The listing builds one solid part. Answer for the finished solid, in the listing's coordinates (mm). Coordinates: 2 decimals unless noted, no trailing zeros. Write each loop counter-clockwise with the first axis right and the second up, starting at its lowest first coordinate (ties: lowest second). Pieces come first, ordered by that corner, then holes.
from build123d import *

# Parameters (mm, degrees)
SKETCH1_R           = 2.38125
BOSS_EXTRUDE1_DEPTH = 5.842
FILLET1_R           = 1.5875
FILLET2_R           = 6.35
FILLET3_R           = 1.5875
CUT_EXTRUDE1_DEPTH  = 122.916897323
FILLET4_R           = 3.175


with BuildPart() as part:
    # Sketch1 → Boss-Extrude1 (new body)
    with BuildSketch(Plane(origin=(0, 0, 0), x_dir=(1, 0, 0), z_dir=(0, 1, 0))):
        Polygon((-10.998522628, -6.35), (-23.207348419, 14.79630657), (-89.198484187, -23.30369343), (-82.848484187, -34.302216058), (-79.673484187, -39.801477372), (-85.172745501, -42.976477372), (-93.847006815, -40.652216058), (-106.547006815, -18.655170802), (-85.725, 40.19630657), (-20.751477372, 61.34261314), (10.998522628, 6.35), align=None)
        with Locations(Location((-28.575, 49.493351826, 0), (0, 0, 270))):
            Circle(SKETCH1_R, mode=Mode.SUBTRACT)
        with Locations(Location((-22.225, 38.494829198, 0), (0, 0, 270))):
            Circle(SKETCH1_R, mode=Mode.SUBTRACT)
        with Locations(Location((-15.875, 27.49630657, 0), (0, 0, 270))):
            Circle(SKETCH1_R, mode=Mode.SUBTRACT)
        with Locations(Location((-9.525, 16.497783942, 0), (0, 0, 270))):
            Circle(SKETCH1_R, mode=Mode.SUBTRACT)
        with Locations(Location((-3.175, 5.499261314, 0), (0, 0, 270))):
            Circle(SKETCH1_R, mode=Mode.SUBTRACT)
        with Locations(Location((-43.2397154, 27.49630657, 0), (0, 0, 270))):
            Circle(SKETCH1_R, mode=Mode.SUBTRACT)
        with Locations(Location((-55.9397154, 27.49630657, 0), (0, 0, 270))):
            Circle(SKETCH1_R, mode=Mode.SUBTRACT)
        with Locations(Location((-68.6397154, 27.49630657, 0), (0, 0, 270))):
            Circle(SKETCH1_R, mode=Mode.SUBTRACT)
        with Locations(Location((-81.3397154, 27.49630657, 0), (0, 0, 270))):
            Circle(SKETCH1_R, mode=Mode.SUBTRACT)
        Polygon((-37.872045256, 40.19630657), (-42.195906773, 47.685454402), (-65.206843197, 40.19630657), align=None, mode=Mode.SUBTRACT)
    extrude(amount=BOSS_EXTRUDE1_DEPTH)

    # Fillet1
    fillet1_edges = [part.edges().sort_by_distance(p)[0] for p in [
        (-42.195906773, 2.921, -47.685454402),
        (-65.206843197, 2.921, -40.19630657),
        (-37.872045256, 2.921, -40.19630657),
    ]]
    fillet(fillet1_edges, radius=FILLET1_R)

    # Fillet2
    fillet2_edges = [part.edges().sort_by_distance(p)[0] for p in [
        (-85.725, 2.921, -40.19630657),
        (-20.751477372, 2.921, -61.34261314),
        (-85.172745501, 2.921, 42.976477372),
        (-93.847006815, 2.921, 40.652216058),
        (-106.547006815, 2.921, 18.655170802),
    ]]
    fillet(fillet2_edges, radius=FILLET2_R)

    # Fillet3
    fillet3_edges = [part.edges().sort_by_distance(p)[0] for p in [
        (10.998522628, 2.921, -6.35),
        (-10.998522628, 2.921, 6.35),
        (-23.207348419, 2.921, -14.79630657),
        (-89.198484187, 2.921, 23.30369343),
        (-79.673484187, 2.921, 39.801477372),
    ]]
    fillet(fillet3_edges, radius=FILLET3_R)

    # Sketch2 → Cut-Extrude1 (cut, through all)
    with BuildSketch(Plane(origin=(0, 5.842, 0), x_dir=(1, 0, 0), z_dir=(0, 1, 0))):
        Polygon((-84.549961559, -5.955170802), (-48.607348419, 14.79630657), (-77.207963999, 14.79630657), align=None)
    extrude(amount=-CUT_EXTRUDE1_DEPTH, mode=Mode.SUBTRACT)

    # Fillet4
    fillet4_edges = [part.edges().sort_by_distance(p)[0] for p in [
        (-84.549961559, 2.921, 5.955170802),
        (-77.207963999, 2.921, -14.79630657),
        (-48.607348419, 2.921, -14.79630657),
    ]]
    fillet(fillet4_edges, radius=FILLET4_R)


solid = part.part
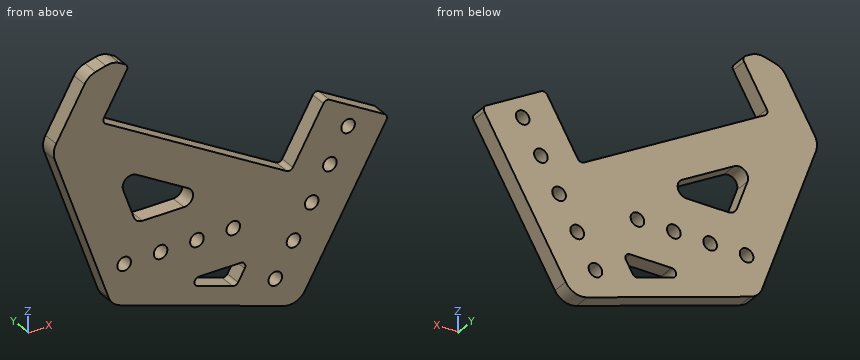
Q1. The part is cut by section C-C, the plane z = -50. Write down the section's boundary in (x, y).
Answers below:
outline: (-55.6, 0) - (-30.9, 0) - (-30.9, 5.84) - (-55.6, 5.84) - close; (-26.25, 0) - (-14.2, 0) - (-14.2, 5.84) - (-26.25, 5.84) - close
Q2. The part is cut by section A-A, the plane x = -63.5. Write down the section's boundary in (y, z).
Answers below:
outline: (0, -47.43) - (5.84, -47.43) - (5.84, -14.8) - (0, -14.8) - close; (0, -6.2) - (5.84, -6.2) - (5.84, 8.47) - (0, 8.47) - close
Q3. Find the intervals of material crossed by probe 1 along X at (y, z) = (2.25, -2); probe 2 along X at (y, z) = (5.05, -5); probe 3 along Z at (x, y) = (-85.5, 0.3), in increasing order.
Answers below:
probe 1: x = -99.24 to -81.73, -70.77 to -45.37, -15.82 to 3.46
probe 2: x = -98.18 to -80.67, -65.58 to -40.18, -17.55 to -5.5, -0.85 to 8.66
probe 3: z = -39.38 to 21.17, 29.71 to 42.49
Q4. The part is cut by section D-D, the plane y = 4.9. State how many separate pieces and enclosed holes the cut face has, then the cut area to 3 significant figures.
Answers below:
separate pieces: 1
enclosed holes: 11
area: 4,980 mm2
Q5. The part is cut by section B-B, the plane z = -28. Write down the section's boundary in (x, y).
Answers below:
outline: (-90.04, 0) - (-83.67, 0) - (-83.67, 5.84) - (-90.04, 5.84) - close; (-79.01, 0) - (-70.97, 0) - (-70.97, 5.84) - (-79.01, 5.84) - close; (-66.31, 0) - (-58.27, 0) - (-58.27, 5.84) - (-66.31, 5.84) - close; (-53.61, 0) - (-45.57, 0) - (-45.57, 5.84) - (-53.61, 5.84) - close; (-40.91, 0) - (-18.2, 0) - (-18.2, 5.84) - (-40.91, 5.84) - close; (-13.55, 0) - (-1.5, 0) - (-1.5, 5.84) - (-13.55, 5.84) - close
Q6. Given pin 1 (3 mm diameter, centred on x = -45, y = 1.5, fed in from -Z); pin 2 (2 mm diameter, centred on x = -90, y = 1, fed in from +Z); pin 3 (1.8 mm diameter, centred on x = -67.5, y = 2, fed in from +Z), each flat-ended and moving along its own axis, determine where each tip first touches the part or whether it passes through.
Answers below:
pin 1: stops at z = -53.94
pin 2: stops at z = 41.95
pin 3: stops at z = 11.3
